```python
from build123d import *

# Parameters (mm, degrees)
F0_R        = 3.175
F1_DEPTH    = 12.7
F2_T1_DEPTH = 95.25
F2_T3_DEPTH = 82.55


# Not quite as in the source:
# - a fillet or chamfer that OpenCascade refuses, or shapes differently, is made with other operations: its cross-section is extruded or revolved along the edge and cut away or added


with BuildPart() as f1:
    # F0 (on Top) → F1 (new body)
    with BuildSketch(Plane.XY):
        with BuildLine():
            Line((23.8110734844, 40.5260987967), (-35.8789265156, 40.5260987967))
            Line((-35.8789265156, 40.5260987967), (-35.8789265156, -16.6239012033))
            Line((-35.8789265156, -16.6239012033), (23.8110734844, -16.6239012033))
            Line((23.8110734844, -16.6239012033), (23.8110734844, -13.4489012033))
            ThreePointArc((23.8110734844, -13.4489012033), (21.5660094542, -12.5189652335), (20.6360734844, -10.2739012033))
            ThreePointArc((20.6360734844, -10.2739012033), (23.8110734844, -7.0989012033), (26.9860734844, -10.2739012033))
            Line((26.9860734844, -10.2739012033), (33.9710734844, -10.2739012033))
            Line((33.9710734844, -10.2739012033), (33.9710734844, 34.1760987967))
            Line((33.9710734844, 34.1760987967), (26.9860734844, 34.1760987967))
            ThreePointArc((26.9860734844, 34.1760987967), (23.8110734844, 31.0010987967), (20.6360734844, 34.1760987967))
            ThreePointArc((20.6360734844, 34.1760987967), (21.5660094542, 36.421162827), (23.8110734844, 37.3510987967))
            Line((23.8110734844, 37.3510987967), (23.8110734844, 40.5260987967))
        make_face()
        with Locations((4.0669361824, -10.2739012033)):
            Circle(F0_R, mode=Mode.SUBTRACT)
        with BuildLine():
            ThreePointArc((10.7640048334, -10.2739012033), (13.9390048334, -7.0989012033), (17.1140048334, -10.2739012033))
            ThreePointArc((17.1140048334, -10.2739012033), (13.9390048334, -13.4489012033), (10.7640048334, -10.2739012033))
        make_face(mode=Mode.SUBTRACT)
        with Locations((2.4716164917, 34.1760987967)):
            Circle(F0_R, mode=Mode.SUBTRACT)
        with BuildLine():
            ThreePointArc((9.966344988, 34.1760987967), (13.141344988, 37.3510987967), (16.316344988, 34.1760987967))
            ThreePointArc((16.316344988, 34.1760987967), (13.141344988, 31.0010987967), (9.966344988, 34.1760987967))
        make_face(mode=Mode.SUBTRACT)
        with BuildLine():
            Line((33.9710734844, 40.5260987967), (23.8110734844, 40.5260987967))
            Line((23.8110734844, 40.5260987967), (23.8110734844, 37.3510987967))
            ThreePointArc((23.8110734844, 37.3510987967), (26.0561375147, 36.421162827), (26.9860734844, 34.1760987967))
            Line((26.9860734844, 34.1760987967), (33.9710734844, 34.1760987967))
            Line((33.9710734844, 34.1760987967), (33.9710734844, 40.5260987967))
        make_face()
        with BuildLine():
            Line((23.8110734844, -13.4489012033), (23.8110734844, -16.6239012033))
            Line((23.8110734844, -16.6239012033), (33.9710734844, -16.6239012033))
            Line((33.9710734844, -16.6239012033), (33.9710734844, -10.2739012033))
            Line((33.9710734844, -10.2739012033), (26.9860734844, -10.2739012033))
            ThreePointArc((26.9860734844, -10.2739012033), (26.0561375147, -12.5189652335), (23.8110734844, -13.4489012033))
        make_face()
    extrude(amount=F1_DEPTH)

    # F2: fillet of radius 5.08 on 4 edges, made by hand

    # F2_s2 → F2_t1 (cut)
    with BuildSketch(Plane.YZ.offset(-48.5789265156)):
        with BuildLine():
            ThreePointArc((-16.6239012033, 5.08), (-15.1360036517, 1.4878975516), (-11.5439012033, 0))
            Line((-11.5439012033, 0), (-16.6239012033, 0))
            Line((-16.6239012033, 0), (-16.6239012033, 5.08))
        make_face()
        with BuildLine():
            ThreePointArc((40.5260987967, 5.08), (39.0382012452, 1.4878975516), (35.4460987967, 0))
            Line((35.4460987967, 0), (40.5260987967, 0))
            Line((40.5260987967, 0), (40.5260987967, 5.08))
        make_face()
    extrude(amount=F2_T1_DEPTH, mode=Mode.SUBTRACT)

    # F2_s4 → F2_t3 (cut)
    with BuildSketch(Plane.XZ.offset(-53.2260987967)):
        with BuildLine():
            ThreePointArc((33.9710734844, 5.08), (32.4831759328, 1.4878975516), (28.8910734844, 0))
            Line((28.8910734844, 0), (33.9710734844, 0))
            Line((33.9710734844, 0), (33.9710734844, 5.08))
        make_face()
        with BuildLine():
            ThreePointArc((-35.8789265156, 5.08), (-34.391028964, 1.4878975516), (-30.7989265156, 0))
            Line((-30.7989265156, 0), (-35.8789265156, 0))
            Line((-35.8789265156, 0), (-35.8789265156, 5.08))
        make_face()
    extrude(amount=F2_T3_DEPTH, mode=Mode.SUBTRACT)


solid = f1.part
```
Work out the finished part from the listing and answer in its coordinate system (mm). Coordinates: 2 decimals unless noted, no trailing zeros. Loops run counter-clockwise (first coordinate to the right, second up) from the corner with the lowest first, then second, coordinate; pieces in that order, holes last. Notation, with made-up numbers: (23.25, 75) -> (62.25, 75) arc R20 cw to (62.25, 93) -> close; hole circle Ø6 at (41.5, -9.75). An arc over 180 degrees is marked (long way). Answer as CSV lines item,"result".
Q1. The part is cut by section C-C on y = -8. Write down the section's boundary in (x, z), and give its area (3 significant figures).
Findings:
outline,"(-35.88, 5.08) arc R5.08 ccw to (-30.8, 0) -> (1.85, 0) -> (1.85, 12.7) -> (-35.88, 12.7) -> close; (6.28, 0) -> (11.72, 0) -> (11.72, 12.7) -> (6.28, 12.7) -> close; (16.15, 0) -> (21.6, 0) -> (21.6, 12.7) -> (16.15, 12.7) -> close; (26.03, 0) -> (28.89, 0) arc R5.08 ccw to (33.97, 5.08) -> (33.97, 12.7) -> (26.03, 12.7) -> close"
area,"707 mm²"
Q2. The part is cut by section A-A on z = 8.25. Write down the section's boundary in (x, y) (3 decimals).
Findings:
outline,"(-35.879, -16.624) -> (33.971, -16.624) -> (33.971, 40.526) -> (-35.879, 40.526) -> close; hole circle Ø6.35 at (2.472, 34.176); hole circle Ø6.35 at (4.067, -10.274); hole circle Ø6.35 at (13.141, 34.176); hole circle Ø6.35 at (13.939, -10.274); hole circle Ø6.35 at (23.811, -10.274); hole circle Ø6.35 at (23.811, 34.176)"
Q3. Find the intervals of material crossed by probe 1 along Y at (x, z) = (22, 2.5); probe 2 along Y at (x, z) = (25.5, 2); probe 3 along X at (y, z) = (-11.5, 6), in increasing order.
Findings:
probe 1,"y = -15.92 to -12.88, -7.67 to 31.57, 36.78 to 39.82"
probe 2,"y = -15.58 to -12.96, -7.59 to 31.49, 36.86 to 39.49"
probe 3,"x = -35.88 to 1.14, 7 to 11.01, 16.87 to 20.88, 26.74 to 33.97"
Q4. The part is cut by section D-D on z = 2.5. Write down the section's boundary in (x, y) (3 decimals).
Findings:
outline,"(-35.175, -15.92) -> (33.267, -15.92) -> (33.267, 39.822) -> (-35.175, 39.822) -> close; hole circle Ø6.35 at (2.472, 34.176); hole circle Ø6.35 at (4.067, -10.274); hole circle Ø6.35 at (13.141, 34.176); hole circle Ø6.35 at (13.939, -10.274); hole circle Ø6.35 at (23.811, -10.274); hole circle Ø6.35 at (23.811, 34.176)"
Q5. For a pull along X with two mould halves and no side action, classify faces 1 (the face through (32.522, 12.351, 1.528)), 2 (the face through (1.783, 31.077, 6.261)), 3 (the face through (-1, -16.624, 9)), 4 (the face through (3.654, -7.126, 6.261)) as +X half, -X half, draft (parallel to the pull), parting line (faces both ways), or undercut.
Findings:
face 1,"+X half"
face 2,"undercut"
face 3,"draft"
face 4,"undercut"
Q6. The part is cut by section B-B on x = -12. Write down the section's boundary in (y, z).
Findings:
outline,"(-16.62, 5.08) arc R5.08 ccw to (-11.54, 0) -> (35.45, 0) arc R5.08 ccw to (40.53, 5.08) -> (40.53, 12.7) -> (-16.62, 12.7) -> close"
